Check sheet for the modelled part. Datum: model origin and axes. Units: mm. Face numbers are marked on the shaded views. Give positions to 0.01 mm unless a question says otherwise; leave off trailing zeros. Order: outer loops, then holes, each group sorted by start corner. A loop starts at its lowest first (then second) coordinate and runs counter-clockwise, first axis right, second up. Notation, with made-up numbers: (65.5, -27.75) -> (72.5, -27.75) arc R18 cw to (72.5, -22.75) -> close; hole circle Ø2 at (-2.75, 22). An arc over 180 degrees is marked (long way). Answer in a Markdown table with one row per item. Add a question column.
(1) Cross-section at C-C (z = 20.5). Record the cut outline in (x, y).
(2) Cross-section at B-B (x = 0). Record the cut outline in (y, z), then the cut area to 3 significant figures.
(3) Release check for a two-part mould opening along Z. For the marked faces 1, 2, 3 and 4 record: released by +Z, released by -Z, zero draft, split by the parting line, or undercut.
(4) Thickness scan on L1, parallel to Y at x = 0, z = 20; L2, parallel to Z at x = -1.5, y = -5.5; L3, parallel to X at y = 5.5, z = 5. Record the ranges inside material, lowest first. Write a range as [from, to].
(5) Cross-section at D-D (z = 35.5). Record the cut outline in (x, y).
(6) Cross-section at A-A (y = 0). Record the cut outline in (x, z).
(7) Go/stop test with flat-tipped pins: pin 1 (2 mm diameter, centred on x = 0, y = 0, fed in from -Z); pin 2 (3.5 mm diameter, centred on y = -2.5, z = 52, fed in from -X). Record where each tip stops, or that it passes through.
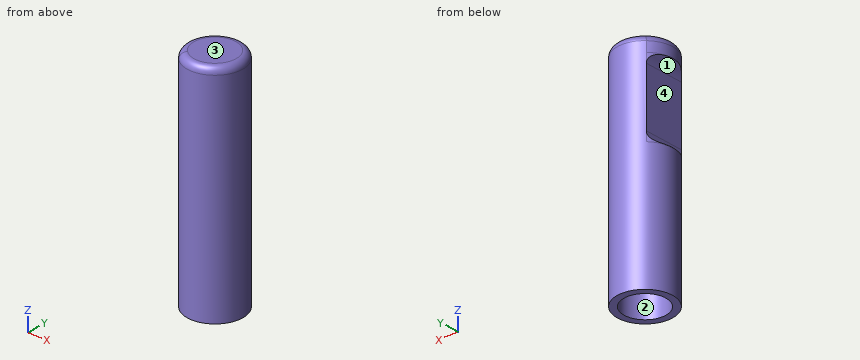
```python
from build123d import *

# Parameters (mm, degrees)
F0_R         = 8.25
F0_R_2       = 6.25
F1_DEPTH     = 34
F2_R         = 8.25
F3_DEPTH     = 32
F5_DEPTH     = 28
F6_DEPTH     = 5
F7_T4_DEPTH  = 26
F7_S5_R      = 8.25
F7_T6_DEPTH  = 15
F7_T10_DEPTH = 26
F7_S11_R     = 8.25
F7_T12_DEPTH = 15
F8_R         = 2


# Not quite as in the source:
# - a fillet or chamfer that OpenCascade refuses, or shapes differently, is made with other operations: its cross-section is extruded or revolved along the edge and cut away or added


with BuildPart() as f1:
    # F0 (on Top) → F1 (new body)
    with BuildSketch(Plane.XY):
        Circle(F0_R)
        Circle(F0_R_2, mode=Mode.SUBTRACT)
    extrude(amount=F1_DEPTH)

    # F2 (on face) → F3 (join)
    with BuildSketch(Plane.XY.offset(34)):
        Circle(F2_R)
    extrude(amount=F3_DEPTH)

    # F4 (on face) → F5 (cut)
    with BuildSketch(Plane.XY.offset(66)):
        with BuildLine():
            Line((-5.6623758265, -6), (-5.6623758265, 6))
            ThreePointArc((-5.6623758265, 6), (-8.25, 0), (-5.6623758265, -6))
        make_face()
    extrude(amount=-F5_DEPTH, mode=Mode.SUBTRACT)

    # F4 (on face) → F6 (join)
    with BuildSketch(Plane.XY.offset(66)):
        with BuildLine():
            Line((-5.6623758265, -6), (-5.6623758265, 6))
            ThreePointArc((-5.6623758265, 6), (-8.25, 0), (-5.6623758265, -6))
        make_face()
    extrude(amount=-F6_DEPTH)

    # F7: fillet of radius 2.8 on 2 edges, made by hand


with BuildPart() as f7_tool2:
    # F7_s3 → F7_t4 (new body)
    with BuildSketch(Plane.XZ.offset(13)):
        with BuildLine():
            ThreePointArc((-8.4623758265, 61), (-6.4824768391, 60.1798989873), (-5.6623758265, 58.2))
            Line((-5.6623758265, 58.2), (-5.6623758265, 61))
            Line((-5.6623758265, 61), (-8.4623758265, 61))
        make_face()
    extrude(amount=-F7_T4_DEPTH)

    # F7_s5 → F7_t6 (intersect, symmetric)
    with BuildSketch(Plane.XY.offset(59.6)):
        Circle(F7_S5_R)
    extrude(amount=F7_T6_DEPTH, both=True, mode=Mode.INTERSECT)


with BuildPart() as f1_1:
    add(f1.part)

    # F7_t1: union F7_tool2
    add(f7_tool2.part)


with BuildPart() as f7_tool8:
    # F7_s9 → F7_t10 (new body)
    with BuildSketch(Plane.XZ.offset(13)):
        with BuildLine():
            ThreePointArc((-8.4623758265, 38), (-6.4824768391, 38.8201010127), (-5.6623758265, 40.8))
            Line((-5.6623758265, 40.8), (-5.6623758265, 38))
            Line((-5.6623758265, 38), (-8.4623758265, 38))
        make_face()
    extrude(amount=-F7_T10_DEPTH)

    # F7_s11 → F7_t12 (intersect, symmetric)
    with BuildSketch(Plane.XY.offset(39.4)):
        Circle(F7_S11_R)
    extrude(amount=F7_T12_DEPTH, both=True, mode=Mode.INTERSECT)


with BuildPart() as f1_2:
    add(f1_1.part)

    # F7_t7: union F7_tool8
    add(f7_tool8.part)

    # F8
    f8_edges = [f1_2.edges().sort_by_distance(p)[0] for p in [
        (-8.25, 0, 66),
    ]]
    fillet(f8_edges, radius=F8_R)


solid = f1_2.part
```
Answer below:
| question | item | result |
|---|---|---|
| 1 | outline | circle Ø16.5 at (0, 0); hole circle Ø12.5 at (0, 0) |
| 2 | outline | (-8.25, 0) -> (-6.25, 0) -> (-6.25, 34) -> (6.25, 34) -> (6.25, 0) -> (8.25, 0) -> (8.25, 64) arc R2 ccw to (6.25, 66) -> (-6.25, 66) arc R2 ccw to (-8.25, 64) -> close |
| 2 | area | 662 mm² |
| 3 | face 1 | undercut |
| 3 | face 2 | zero draft |
| 3 | face 3 | released by +Z |
| 3 | face 4 | undercut |
| 4 | L1 | y = [-8.25, -6.25], [6.25, 8.25] |
| 4 | L2 | z = [34, 66] |
| 4 | L3 | x = [-6.15, -2.97], [2.97, 6.15] |
| 5 | outline | circle Ø16.5 at (0, 0) |
| 6 | outline | (-8.25, 0) -> (-6.25, 0) -> (-6.25, 34) -> (6.25, 34) -> (6.25, 0) -> (8.25, 0) -> (8.25, 64) arc R2 ccw to (6.25, 66) -> (-6.25, 66) arc R2 ccw to (-8.25, 64) -> (-8.25, 60.99) arc R2.8 cw to (-5.66, 58.2) -> (-5.66, 40.8) arc R2.8 cw to (-8.25, 38.01) -> close |
| 7 | pin 1 | stops at z = 34 |
| 7 | pin 2 | stops at x = -5.66 |
